from build123d import *

# Parameters (mm, degrees)
SKETCH1_R           = 2.25
BOSS_EXTRUDE1_DEPTH = 3.175


with BuildPart() as part:
    # Sketch1 → Boss-Extrude1 (new body)
    with BuildSketch(Plane.XY):
        Polygon((-133.35, -88.9), (177.8, -88.9), (177.8, 3.175), (133.35, 3.175), (133.35, 22.225), (177.8, 22.225), (177.8, 88.9), (-177.8, 88.9), (-177.8, -31.75), (-133.35, -31.75), align=None)
        with Locations((-149.225, -22.225)):
            Circle(SKETCH1_R, mode=Mode.SUBTRACT)
        with Locations((95.25, -73.025)):
            Circle(SKETCH1_R, mode=Mode.SUBTRACT)
        with Locations((95.25, -42.545)):
            Circle(SKETCH1_R, mode=Mode.SUBTRACT)
        with Locations((149.225, -22.225)):
            Circle(SKETCH1_R, mode=Mode.SUBTRACT)
        with Locations((-149.225, 49.2125)):
            Circle(SKETCH1_R, mode=Mode.SUBTRACT)
        with Locations((149.225, 49.2125)):
            Circle(SKETCH1_R, mode=Mode.SUBTRACT)
    extrude(amount=-BOSS_EXTRUDE1_DEPTH)


solid = part.part
Geometry: final body of the model. Coordinates: model frame, mm. Give positions to 0.01 mm unless a question says otherwise; leave off trailing zeros. Write each loop counter-clockwise with the first axis right and the second up, starting at its lowest first coordinate (ties: lowest second). Pieces come first, ordered by that corner, then holes.
(1) Cut plane A-A, the plane z = -1.35. Give the number of separate pieces and of enclosed holes in the cut face, then the cut area to 3 significant figures.
(2) Cut plane B-B, the plane y = -62.5. Return loops of the section in (x, z) (3 decimals).
(3) First-contact query: P1, Ø1.6, axis at y = -57, z = -1.5, coming from the -X side; P2, Ø1.6, axis at x = -165.5, z = -1, coming from the -Y side. Flat tips, straight axial feed; report the tip coordinate or a pass-through.
(4) Ray query, line 1 (X direction, y = -45, z = -2.05); line 2 (Y direction, x = -158.5, z = -0.55); line 3 (Y direction, x = 136.5, z = -2.95) (3 decimals). Return the intervals inside material, ascending.
Values follow:
1. separate pieces: 1
1. enclosed holes: 6
1. area: 59,700 mm2
2. outline: (-133.35, -3.175) - (177.8, -3.175) - (177.8, 0) - (-133.35, 0) - close
3. P1: stops at x = -133.35
3. P2: stops at y = -31.75
4. line 1: x = -133.35 to 177.8
4. line 2: y = -31.75 to 88.9
4. line 3: y = -88.9 to 3.175, 22.225 to 88.9
